```python
from build123d import *

# Parameters (mm, degrees)
SKETCH_1_R          = 23
EXTRUDE_1_DEPTH     = 2
SKETCH_2_R          = 1.6
SKETCH_2_R_2        = 7.5
CUT_EXTRUDE_1_DEPTH = 33.588341474


with BuildPart() as part:
    # ｽｹｯﾁ1 → ﾎﾞｽ - 押し出し1 (new body)
    with BuildSketch(Plane.XY):
        Circle(SKETCH_1_R)
    extrude(amount=EXTRUDE_1_DEPTH)

    # ｽｹｯﾁ2 → ｶｯﾄ - 押し出し1 (cut, through all)
    with BuildSketch(Plane.XY.offset(2)):
        with Locations((-3.5, 17.656443583)):
            Circle(SKETCH_2_R)
        with Locations((3.5, 17.656443583)):
            Circle(SKETCH_2_R)
        with Locations((13.540928683, 11.859310705)):
            Circle(SKETCH_2_R)
        with Locations((17.040928683, 5.797132878)):
            Circle(SKETCH_2_R)
        with Locations((17.040928683, -5.797132878)):
            Circle(SKETCH_2_R)
        with Locations((13.540928683, -11.859310705)):
            Circle(SKETCH_2_R)
        with Locations((3.5, -17.656443583)):
            Circle(SKETCH_2_R)
        with Locations((-3.5, -17.656443583)):
            Circle(SKETCH_2_R)
        with Locations((-13.540928683, -11.859310705)):
            Circle(SKETCH_2_R)
        with Locations((-17.040928683, -5.797132878)):
            Circle(SKETCH_2_R)
        with Locations((-17.040928683, 5.797132878)):
            Circle(SKETCH_2_R)
        with Locations((-13.540928683, 11.859310705)):
            Circle(SKETCH_2_R)
        Circle(SKETCH_2_R_2)
        with Locations((0, 11.5)):
            Circle(SKETCH_2_R)
        with Locations((-9.959292144, -5.75)):
            Circle(SKETCH_2_R)
        with Locations((9.959292144, -5.75)):
            Circle(SKETCH_2_R)
    extrude(amount=-CUT_EXTRUDE_1_DEPTH, mode=Mode.SUBTRACT)


solid = part.part
```
Geometry check sheet. Reference: the model listing, model coordinates, mm. Coordinates: 2 decimals unless noted, no trailing zeros. Order: outer loops, then holes, each group sorted by start corner. A loop starts at its lowest first (then second) coordinate and runs counter-clockwise, first axis right, second up. Notation, with made-up numbers: (64, 62.5) - (91, 62.5) arc R28 cw to (91, 91.5) - close; hole circle Ø5 at (51.25, -28). An arc over 180 degrees is marked (long way). Answer in a Markdown table with one row per item. Add a question column.
1. Draft check along Y on faces 1 (the face through (-7.493, 0.33, 1.014)), 2 (the face through (-2.994, 22.804, 0.986)), 3 (the face through (-5.43, 5.43, 0)). Enter one of: +Y half, -Y half, draft (parallel to the pull), parting line (faces both ways), or undercut.
2. Section check B-B (y = -1). Enter the section's corners in (x, z), plus the area to 3 significant figures.
3. Section check D-D (x = 9.5). Enter the section's corners in (y, z).
4. Section check C-C (z = 0.5). Give the number of separate pieces and of enclosed holes in the cut face, plus the area to 3 significant figures.
5. Gauge pin test, flat end, axial feed: pin 1 Ø1 at (x, z) = (-7, 0.5) entering from +Y. Record the tip position at first contact, or that the pin passes through.
6. Section check A-A (x = 0). Enter the section's corners in (y, z).
7. Material ranges on L1, parallel to Y at x = 0, z = 0.45; L2, parallel to Y at x = -15, z = 0.65; L3, parallel to X at y = 10.5, z = 0.2, recorded low to high. Write a range as [from, to].
Data:
| question | item | result |
|---|---|---|
| 1 | face 1 | undercut |
| 1 | face 2 | parting line |
| 1 | face 3 | draft |
| 2 | outline | (-22.98, 0) - (-7.43, 0) - (-7.43, 2) - (-22.98, 2) - close; (7.43, 0) - (22.98, 0) - (22.98, 2) - (7.43, 2) - close |
| 2 | area | 62.2 mm² |
| 3 | outline | (-20.95, 0) - (-7.28, 0) - (-7.28, 2) - (-20.95, 2) - close; (-4.22, 0) - (20.95, 0) - (20.95, 2) - (-4.22, 2) - close |
| 4 | separate pieces | 1 |
| 4 | enclosed holes | 16 |
| 4 | area | 1,360 mm² |
| 5 | pin 1 | stops at y = 22.06 |
| 6 | outline | (-23, 0) - (-7.5, 0) - (-7.5, 2) - (-23, 2) - close; (7.5, 0) - (9.9, 0) - (9.9, 2) - (7.5, 2) - close; (13.1, 0) - (23, 0) - (23, 2) - (13.1, 2) - close |
| 7 | L1 | y = [-23, -7.5], [7.5, 9.9], [13.1, 23] |
| 7 | L2 | y = [-17.44, -12.52], [-11.2, 11.2], [12.52, 17.44] |
| 7 | L3 | x = [-20.46, -14.38], [-12.7, -1.25], [1.25, 12.7], [14.38, 20.46] |
